```python
from build123d import *

# Parameters (mm, degrees)
F0_W     = 150
F0_H     = 150
F0_W_2   = 100
F0_H_2   = 100
F1_DEPTH = 5
F2_SIZE  = 25
F4_D     = 4


with BuildPart() as f1:
    # F0 (on Front) → F1 (new body)
    with BuildSketch(Plane.XZ):
        Rectangle(F0_W, F0_H)
        Rectangle(F0_W_2, F0_H_2, mode=Mode.SUBTRACT)
    extrude(amount=F1_DEPTH)

    # F2
    f2_edges = [f1.edges().sort_by_distance(p)[0] for p in [
        (-75, -2.5, 75),
        (75, -2.5, 75),
        (-75, -2.5, -75),
        (75, -2.5, -75),
    ]]
    chamfer(f2_edges, length=F2_SIZE)

    # F4 (through all)
    with Locations(Plane.XZ.offset(5)):
        with Locations((56, 56), (56, -56), (-52.823993, -56), (-56, 56)):
            Hole(F4_D / 2)


solid = f1.part
```
Verification items for the finished model (mm, model axes). A direction names the side the tool comes from. Give positions to 0.01 mm unless a question says otherwise; leave off trailing zeros. Order: outer loops, then holes, each group sorted by start corner. A loop starts at its lowest first (then second) coordinate and runs counter-clockwise, first axis right, second up. Notation, with made-up numbers: M -9.5,56 L 33.5,56 A23 cw 33.5,86 Z; hole C 71,-30.5 d5. An arc over 180 degrees is marked long. Return JSON: item names as keys, results as strings. Group by question number.
1) Go/stop test with a flat-tipped pin: pin 1 Ø3.5 at (x, z) = (-52.82, -56) entering from +Y. Record where the tip stops, or that it passes through.
2) Mould release check, pull along Z, two halves, no side actions. Record for faces 1 (the face through (-62, -2, 63)), 2 (the face through (-1, -2, -75)), 3 (the face through (50, -2, -1)): pulls with the +Z half, pulls with the -Z half, needs draft (parallel to the pull), parting line crosses it, or undercut.
3) Scan lines: line 1 (X direction, y = -2.1, z = -16); line 2 (Z direction, x = 56, y = -3.2). Record each from-to range of solid material in increasing order.
4) Section check D-D on y = -1.7. Record the cut outline in (x, z), and give its area (3 significant figures).
5) Access from +Z, -Z, +X, -X, +Y, -Y to the whole of each face (thin tool, end or side, straight path). Record for faces 4 (the face through (-62, -2, -63)), 5 (the face through (-1, -2, -50)).
6) Section check A-A on x = 56. Record the cut outline in (y, z).
7) Section check C-C on x = -11. Record the cut outline in (y, z).
8) Section check B-B on z = -56. Record the cut outline in (x, y).
Answer block:
{
 "1": {"pin 1": "passes through"},
 "2": {"face 1": "pulls with the +Z half", "face 2": "pulls with the -Z half", "face 3": "undercut"},
 "3": {"line 1": "x = -75 to -50, 50 to 75", "line 2": "z = -69 to -58, -54 to 54, 58 to 69"},
 "4": {"outline": "M -75,-50 L -50,-75 L 50,-75 L 75,-50 L 75,50 L 50,75 L -50,75 L -75,50 Z; hole C -56,56 d4; hole C -52.82,-56 d4; hole M -50,-50 L 50,-50 L 50,50 L -50,50 Z; hole C 56,-56 d4; hole C 56,56 d4", "area": "11,200 mm^2"},
 "5": {"face 4": "-Z, -X, +Y, -Y", "face 5": "+Y, -Y"},
 "6": {"outline": "M -5,-69 L 0,-69 L 0,-58 L -5,-58 Z; M -5,-54 L 0,-54 L 0,54 L -5,54 Z; M -5,58 L 0,58 L 0,69 L -5,69 Z"},
 "7": {"outline": "M -5,-75 L 0,-75 L 0,-50 L -5,-50 Z; M -5,50 L 0,50 L 0,75 L -5,75 Z"},
 "8": {"outline": "M -69,-5 L -54.82,-5 L -54.82,0 L -69,0 Z; M -50.82,-5 L 54,-5 L 54,0 L -50.82,0 Z; M 58,-5 L 69,-5 L 69,0 L 58,0 Z"}
}
